For this review, take the finished solid that the model builds, in its own axes (mm). Face numbers are marked on the shaded views. Give positions to 0.01 mm unless a question says otherwise; leave off trailing zeros. Loops run counter-clockwise (first coordinate to the right, second up) from the corner with the lowest first, then second, coordinate; pieces in that order, holes last. Notation, with made-up numbers: M -17.5,42.25 L 37.5,42.25 A19 cw 37.5,74.25 Z; hole C 10,65 d5. An arc over 180 degrees is marked long. Use CSV: the item, a comma, the result in double quotes. Start each with the question number.
1. To check wall thickness, follow line 1 (Z direction, x = 3, y = -38); line 2 (Y direction, x = -4.5, z = 282); line 3 (Z direction, x = 5, y = -70.5). State the ranges of each line that lie inside material, in increasing order. Write a range as [from, to].
2. Take a section at A-A, the plane x = -6. Write out the cut boundary in (y, z), and give its area (3 significant figures).
3. Insertion check: P1, Ø5, axis at x = -6.5, y = -45.5, coming from the +Z side; P2, Ø5, axis at x = -7, y = -66.5, coming from the +Z side; P3, Ø3, axis at x = -0.5, y = -41.5, coming from the -Z side; P4, Ø9.5, axis at y = -52.98, z = 284.71, coming from the +X side. Each pin has a flat end and moves straight along its axis. Give the tip position at first contact, or say it passes through.
4. Take a section at B-B, the plane x = -8.75. Write out the cut boundary in (y, z), and give its area (3 significant figures).
5. The part is to be moulded in two halves that separate along Y. For the marked faces 1, 2 and 3, say which applies: pulls with the +Y half, pulls with the -Y half, needs draft (parallel to the pull), parting line crosses it, or undercut.
from build123d import *

# Parameters (mm, degrees)
SKETCH5_R      = 2
EXTRUDE4_DEPTH = 100
SKETCH6_R      = 3
EXTRUDE5_DEPTH = 100


with BuildPart() as part:
    # Fillet4: read off the stored shape, not the designer's step
    # Fillet4 outline → Fillet4 (revolve)
    with BuildSketch(Plane(origin=(0, -52.981969609, 284.712869435), x_dir=(0, 1, 0), z_dir=(0, 0, -1))):
        with BuildLine():
            Line((25, -5), (25, 5))
            ThreePointArc((25, 5), (23.535533906, 8.535533906), (20, 10))
            Line((20, 10), (0, 10))
            Line((0, 10), (0, -10))
            Line((0, -10), (20, -10))
            ThreePointArc((20, -10), (23.535533906, -8.535533906), (25, -5))
        make_face()
    revolve(axis=Axis((0, -52.981969609, 284.712869435), (1, 0, 0)))

    # Sketch5 → Extrude4 (cut)
    with BuildSketch(Plane(origin=(10, 0, 0), x_dir=(0, 0, -1), z_dir=(1, 0, 0))):
        with Locations((-284.712869435, -52.981969609)):
            Circle(SKETCH5_R)
    extrude(amount=-EXTRUDE4_DEPTH, mode=Mode.SUBTRACT)

    # Sketch6 → Extrude5 (cut)
    with BuildSketch(Plane(origin=(10, 0, 0), x_dir=(0, 0, -1), z_dir=(1, 0, 0))):
        with Locations((-284.712869435, -52.981969609)):
            Circle(SKETCH6_R)
    extrude(amount=-EXTRUDE5_DEPTH, mode=Mode.SUBTRACT)


solid = part.part
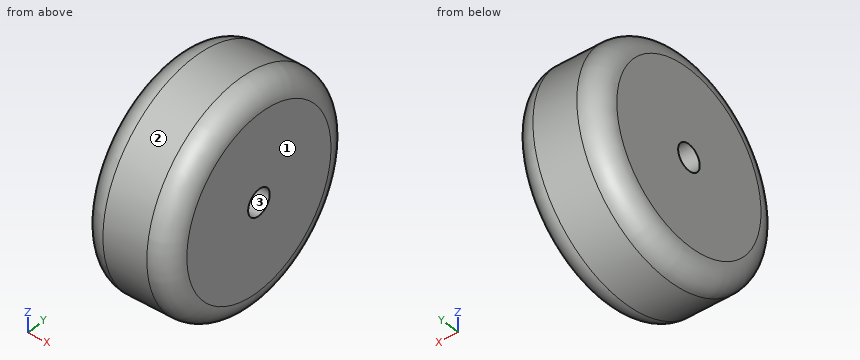
Result set:
1,line 1,"[264.7, 304.73]"
1,line 2,"[-77.83, -54.26], [-51.7, -28.13]"
1,line 3,"[266.88, 302.55]"
2,outline,"C -52.98,284.71 d49.8; hole C -52.98,284.71 d6"
2,area,"1,920 mm2"
3,P1,"z = 309.14"
3,P2,"z = 306.94"
3,P3,"z = 261.79"
3,P4,"x = 10"
4,outline,"C -52.98,284.71 d46.61; hole C -52.98,284.71 d6"
4,area,"1,680 mm2"
5,face 1,"needs draft"
5,face 2,"parting line crosses it"
5,face 3,"undercut"
